from build123d import *

# Parameters (mm, degrees)
EXTRUDE_1_DEPTH             = 90
SKETCH_2_W                  = 90
SKETCH_2_H                  = 17.75
EXTRUDE_2_DEPTH             = 8.2
SKETCH_3_W                  = 90
SKETCH_3_H                  = 50.95
EXTRUDE_3_DEPTH             = 8.2
SKETCH_4_W                  = 3.95
SKETCH_4_H                  = 29.5
CUT_EXTRUDE_1_DEPTH         = 96.44153315
SKETCH_5_W                  = 3.95
SKETCH_5_H                  = 6.2
CUT_EXTRUDE_2_DEPTH         = 96.44153315
SKETCH_6_W                  = 2.25
SKETCH_6_H                  = 3.95
CUT_EXTRUDE_3_DEPTH         = 96.44153315
SKETCH_7_W                  = 4.5
SKETCH_7_H                  = 3.95
CUT_EXTRUDE_4_DEPTH         = 96.44153315
SKETCH_8_W                  = 2.25
SKETCH_8_H                  = 3.95
CUT_EXTRUDE_5_DEPTH         = 96.44153315
SKETCH_9_W                  = 3.95
SKETCH_9_H                  = 2.25
CUT_EXTRUDE_6_DEPTH         = 96.44153315
SKETCH_10_W                 = 20.2
SKETCH_10_H                 = 45.2
CUT_EXTRUDE_7_DEPTH         = 86
HOLE_WIZARD_2_5_2_5_1_D     = 2.5
HOLE_WIZARD_4_5_4_5_1_D     = 4.5
HOLE_WIZARD_8_3_8_3_1_D     = 8.3
HOLE_WIZARD_8_3_8_3_1_DEPTH = 3.2
FILLET_1_R                  = 2
FILLET_2_R                  = 2
EXTRUDE_START               = -90
SKETCH_17_R                 = 1.25
EXTRUDE_4_DEPTH             = 90
CUT_EXTRUDE_START           = -100
SKETCH_18_R                 = 4.15
CUT_EXTRUDE_8_DEPTH         = 100
CUT_EXTRUDE_9_DEPTH         = 106
SKETCH_20_W                 = 90
SKETCH_20_H                 = 22.108571968
EXTRUDE_5_DEPTH             = 2


with BuildPart() as part:
    # Эскиз1 → Бобышка-Вытянуть1 (new body)
    with BuildSketch(Plane(origin=(90, 0, 0), x_dir=(0, 0, -1), z_dir=(1, 0, 0))):
        with BuildLine():
            Line((6.75, -24.093761792), (6.75, 19.25))
            Line((6.75, 19.25), (-11.593761792, 19.25))
            ThreePointArc((-11.593761792, 19.25), (-15.325, 18), (-11.593761792, 16.75))
            Line((-11.593761792, 16.75), (-11, 16.75))
            Line((-11, 16.75), (-11, -16.75))
            Line((-11, -16.75), (-11.593761792, -16.75))
            ThreePointArc((-11.593761792, -16.75), (-15.325, -18), (-11.593761792, -19.25))
            Line((-11.593761792, -19.25), (-11, -19.25))
            Line((-11, -19.25), (-11, -23.5))
            Line((-11, -23.5), (-6.75, -23.5))
            Line((-6.75, -23.5), (-6.75, -24.093761792))
            ThreePointArc((-6.75, -24.093761792), (-5.5, -27.825), (-4.25, -24.093761792))
            Line((-4.25, -24.093761792), (-4.25, -23.5))
            Line((-4.25, -23.5), (4.25, -23.5))
            Line((4.25, -23.5), (4.25, -24.093761792))
            ThreePointArc((4.25, -24.093761792), (5.5, -27.825), (6.75, -24.093761792))
        make_face()
    extrude(amount=-EXTRUDE_1_DEPTH)

    # Эскиз2 → Бобышка-Вытянуть2 (add)
    with BuildSketch(Plane(origin=(0, 19.25, 0), x_dir=(-1, 0, 0), z_dir=(0, 1, 0))):
        with Locations((-45, 2.125)):
            Rectangle(SKETCH_2_W, SKETCH_2_H)
    extrude(amount=EXTRUDE_2_DEPTH)

    # Эскиз3 → Бобышка-Вытянуть3 (add)
    with BuildSketch(Plane(origin=(0, 0, -6.75), x_dir=(-1, 0, 0), z_dir=(0, 0, -1))):
        with Locations((-45, 1.975)):
            Rectangle(SKETCH_3_W, SKETCH_3_H)
    extrude(amount=EXTRUDE_3_DEPTH)

    # Эскиз4 → Вырез-Вытянуть1 (cut, through all)
    with BuildSketch(Plane.ZY):
        with Locations((-12.975, 0)):
            Rectangle(SKETCH_4_W, SKETCH_4_H)
    extrude(amount=-CUT_EXTRUDE_1_DEPTH, mode=Mode.SUBTRACT)

    # Эскиз5 → Вырез-Вытянуть2 (cut, through all)
    with BuildSketch(Plane.ZY):
        with Locations((-12.975, 24.35)):
            Rectangle(SKETCH_5_W, SKETCH_5_H)
    extrude(amount=-CUT_EXTRUDE_2_DEPTH, mode=Mode.SUBTRACT)

    # Эскиз6 → Вырез-Вытянуть3 (cut, through all)
    with BuildSketch(Plane.ZY):
        with Locations((-9.875, 25.475)):
            Rectangle(SKETCH_6_W, SKETCH_6_H)
    extrude(amount=-CUT_EXTRUDE_3_DEPTH, mode=Mode.SUBTRACT)

    # Эскиз7 → Вырез-Вытянуть4 (cut, through all)
    with BuildSketch(Plane.ZY):
        with Locations((0, 25.475)):
            Rectangle(SKETCH_7_W, SKETCH_7_H)
    extrude(amount=-CUT_EXTRUDE_4_DEPTH, mode=Mode.SUBTRACT)

    # Эскиз8 → Вырез-Вытянуть5 (cut, through all)
    with BuildSketch(Plane.ZY):
        with Locations((9.875, 25.475)):
            Rectangle(SKETCH_8_W, SKETCH_8_H)
    extrude(amount=-CUT_EXTRUDE_5_DEPTH, mode=Mode.SUBTRACT)

    # Эскиз9 → Вырез-Вытянуть6 (cut, through all)
    with BuildSketch(Plane.ZY):
        with Locations((-12.975, -22.375)):
            Rectangle(SKETCH_9_W, SKETCH_9_H)
    extrude(amount=-CUT_EXTRUDE_6_DEPTH, mode=Mode.SUBTRACT)

    # Эскиз10 → Вырез-Вытянуть7 (cut)
    with BuildSketch(Plane(origin=(90, 0, 0), x_dir=(0, 0, -1), z_dir=(1, 0, 0))):
        Rectangle(SKETCH_10_W, SKETCH_10_H)
    extrude(amount=-CUT_EXTRUDE_7_DEPTH, mode=Mode.SUBTRACT)

    # Диаметр отверстия Ø2.5 (2.5)1 (through all)
    with Locations(Plane(origin=(90, 0, 0), x_dir=(0, 0, -1), z_dir=(1, 0, 0))):
        with Locations((5.5, -25.75), (-13.25, -18), (-5.5, -25.75), (-13.25, 18)):
            Hole(HOLE_WIZARD_2_5_2_5_1_D / 2)

    # Диаметр отверстия Ø4.5 (4.5)1 (through all)
    with Locations(Plane.ZY):
        with Locations((-13.25, -18), (-13.25, 18), (-5.5, 25.75), (5.5, 25.75)):
            Hole(HOLE_WIZARD_4_5_4_5_1_D / 2)

    # Диаметр отверстия Ø8.3 (8.3)1
    with Locations(Plane.ZY):
        with Locations((0, 0)):
            Hole(HOLE_WIZARD_8_3_8_3_1_D / 2, depth=HOLE_WIZARD_8_3_8_3_1_DEPTH)

    # Скругление1
    fillet_1_edges = [part.edges().sort_by_distance(p)[0] for p in [
        (45, 23.5, 8.75),
    ]]
    fillet(fillet_1_edges, radius=FILLET_1_R)

    # Скругление2
    fillet_2_edges = [part.edges().sort_by_distance(p)[0] for p in [
        (45, 23.5, -8.75),
        (45, 23.5, 2.25),
        (45, 23.5, -2.25),
        (45, -21.25, -11),
        (4, 0, -10.1),
        (4, -22.6, 0),
        (4, 0, 10.1),
        (4, 22.6, 0),
        (45, 14.75, -11),
        (45, -14.75, -11),
        (45, 21.25, -11),
    ]]
    fillet(fillet_2_edges, radius=FILLET_2_R)

    # Эскиз17 → Бобышка-Вытянуть4 (add)
    with BuildSketch(Plane(origin=(90, 0, 0), x_dir=(0, 0, -1), z_dir=(1, 0, 0)).offset(EXTRUDE_START)):
        with Locations((5.5, -25.75)):
            Circle(SKETCH_17_R)
        with Locations((-5.5, -25.75)):
            Circle(SKETCH_17_R)
        with Locations((-13.25, -18)):
            Circle(SKETCH_17_R)
        with Locations((-13.25, 18)):
            Circle(SKETCH_17_R)
    extrude(amount=EXTRUDE_4_DEPTH)

    # Эскиз18 → Вырез-Вытянуть8 (cut)
    with BuildSketch(Plane.ZY.offset(CUT_EXTRUDE_START)):
        Circle(SKETCH_18_R)
    extrude(amount=CUT_EXTRUDE_8_DEPTH, mode=Mode.SUBTRACT)

    # Эскиз19 → Вырез-Вытянуть9 (cut)
    with BuildSketch(Plane(origin=(90, 0, 0), x_dir=(0, 0, -1), z_dir=(1, 0, 0))):
        Polygon((10.1, -22.6), (-10.1, -22.6), (-27.028488592, -22.6), (-27.028488592, 40.291612525), (29.6277603, 40.291612525), (29.6277603, -22.6), align=None)
    extrude(amount=-CUT_EXTRUDE_9_DEPTH, mode=Mode.SUBTRACT)

    # Эскиз20 → Бобышка-Вытянуть5 (add)
    with BuildSketch(Plane(origin=(0, -22.6, 0), x_dir=(1, 0, 0), z_dir=(0, 1, 0))):
        with Locations((45, 0.054285984)):
            Rectangle(SKETCH_20_W, SKETCH_20_H)
    extrude(amount=EXTRUDE_5_DEPTH)


solid = part.part
Read the model definition and answer for the solid it produces. Units are mm, in the model's axes. A direction names the side the tool comes from. Coordinates: 2 decimals unless noted, no trailing zeros. Order: outer loops, then holes, each group sorted by start corner. A loop starts at its lowest first (then second) coordinate and runs counter-clockwise, first axis right, second up. Notation, with made-up numbers: (-13.5, -19) -> (-5.5, -19) arc R10 ccw to (-5.5, -14) -> close; hole circle Ø11 at (61, -18). An arc over 180 degrees is marked (long way). Answer as a JSON object with one key per item and string values.
1) The mould has two halves that part along Z. Classify faces 3 (the face through (46, -23.5, -9)), 4 (the face through (45.63, -27.824, -5.428)), 5 (the face through (46, -23.5, 0)), 6 (the face through (44, -22, 11)): released by +Z, released by -Z, zero draft, split by the parting line, or undercut.
Model answer:
{"face 3": "zero draft", "face 4": "undercut", "face 5": "undercut", "face 6": "released by +Z"}
2) Consider line 1 along Y through (x, z) = (67, 0.25); line 2 along Z through (x, y) = (9, -25.75) (3 decimals); line 3 along Y through (x, z) = (26.5, -4). Determine where each line is inside the solid, lowest interval first. Write a range as from..to.
Model answer:
{"line 1": "y = -23.5..-20.6", "line 2": "z = -7.575..-3.425, 3.425..7.575", "line 3": "y = -27.18..-24.32, -23.5..-20.6"}
3) A cutting plane is placed at B-B, the plane x = 39. Determine the outline of the cut face in (y, z) (3 decimals).
Model answer:
{"outline": "(-24.094, -6.75) -> (-23.5, -6.75) -> (-23.5, -11) -> (-23.25, -11) arc R2 cw to (-22.6, -11.109) -> (-20.6, -11.109) -> (-20.6, 11) -> (-23.5, 11) -> (-23.5, 6.75) -> (-24.094, 6.75) arc R2.075 ccw (long way) to (-24.094, 4.25) -> (-23.5, 4.25) -> (-23.5, -4.25) -> (-24.094, -4.25) arc R2.075 ccw (long way) to start"}
4) A cutting plane is placed at A-A, the plane y = -25.75. Determine the outline of the cut face in (x, z) (3 decimals), plus the area to 3 significant figures.
Model answer:
{"outline": "(0, -7.575) -> (90, -7.575) -> (90, -3.425) -> (0, -3.425) -> close; (0, 3.425) -> (90, 3.425) -> (90, 7.575) -> (0, 7.575) -> close", "area": "747 mm²"}
5) A tool of negligible diameter and unlimited length cuts with its end or side. For faces 1 (the face through (46, -23.5, 9)), 2 (the face through (0, -23, 0)), from which of +Z, -Z, +X, -X, +Y, -Y can it reach the whole face along a straight path? Write none if from no direction.
Model answer:
{"face 1": "+Z, +X, -X", "face 2": "+Z, -Z, -X, +Y, -Y"}
6) Each of these flat-tipped pins is pushed along its axis until it touches: pin 1 (3.5 mm diameter, centred on x = 59, z = -9, fed in from -Y); pin 2 (0.5 mm diameter, centred on x = 51, y = -24, fed in from +Z); pin 3 (4 mm diameter, centred on x = 62, z = 2, fed in from -Y). Where does it stop, or does it pass through?
Model answer:
{"pin 1": "stops at y = -26.86", "pin 2": "stops at z = 6.93", "pin 3": "stops at y = -27.18"}
